from build123d import *

# Parameters (mm, degrees)
SKETCH_W        = 193
SKETCH_H        = 50
PAD_DEPTH       = 1.5
SKETCH001_W     = 193
SKETCH001_H     = 50
SKETCH001_W_2   = 190
SKETCH001_H_2   = 47.5
PAD001_DEPTH    = 28.5
SKETCH002_W     = 8
SKETCH002_H     = 6.75
PAD002_DEPTH    = 2
SKETCH003_R     = 3
PAD003_DEPTH    = 14.5
SKETCH004_R     = 2
POCKET_DEPTH    = 5
SKETCH005_W     = 13.4
SKETCH005_H     = 12
POCKET001_DEPTH = 5


with BuildPart() as part:
    # Sketch → Pad (new body)
    with BuildSketch(Plane.XY):
        with Locations((96.5, 25)):
            Rectangle(SKETCH_W, SKETCH_H)
    extrude(amount=PAD_DEPTH)

    # Sketch001 (on Face6 of Pad) → Pad001 (join)
    with BuildSketch(Plane.XY.offset(1.5)):
        with Locations((96.5, 25)):
            Rectangle(SKETCH001_W, SKETCH001_H)
        with Locations((96.5, 25)):
            Rectangle(SKETCH001_W_2, SKETCH001_H_2, mode=Mode.SUBTRACT)
    extrude(amount=PAD001_DEPTH)

    # Sketch002 (on Face15 of Pad001) → Pad002 (join)
    with BuildSketch(Plane.XY.offset(1.5)):
        with Locations((5.5, 45.375)):
            Rectangle(SKETCH002_W, SKETCH002_H)
        with Locations((187.5, 45.375)):
            Rectangle(SKETCH002_W, SKETCH002_H)
        with Locations((187.5, 4.625)):
            Rectangle(SKETCH002_W, SKETCH002_H)
        with Locations((5.5, 4.625)):
            Rectangle(SKETCH002_W, SKETCH002_H)
    extrude(amount=PAD002_DEPTH)

    # Sketch003 (on Face19 of Pad002) → Pad003 (join)
    with BuildSketch(Plane.XY.offset(3.5)):
        with Locations((5.5, 46)):
            Circle(SKETCH003_R)
        with Locations((5.5, 4)):
            Circle(SKETCH003_R)
        with Locations((187.5, 46)):
            Circle(SKETCH003_R)
        with Locations((187.5, 4)):
            Circle(SKETCH003_R)
    extrude(amount=PAD003_DEPTH)

    # Sketch004 (on Face24 of Pad003) → Pocket (cut)
    with BuildSketch(Plane.XY.offset(18)):
        with Locations((187.5, 46)):
            Circle(SKETCH004_R)
        with Locations((187.5, 4)):
            Circle(SKETCH004_R)
        with Locations((5.5, 46)):
            Circle(SKETCH004_R)
        with Locations((5.5, 4)):
            Circle(SKETCH004_R)
    extrude(amount=-POCKET_DEPTH, mode=Mode.SUBTRACT)

    # Sketch005 (on Face7 of Pocket) → Pocket001 (cut)
    with BuildSketch(Plane(origin=(0, 0, 0), x_dir=(0, -1, 0), z_dir=(-1, 0, 0))):
        with Locations((-25, 13.5)):
            Rectangle(SKETCH005_W, SKETCH005_H)
    extrude(amount=-POCKET001_DEPTH, mode=Mode.SUBTRACT)


solid = part.part
The model under review builds one solid part; all positions refer to its coordinate system, in mm. A direction names the side the tool comes from. Round coordinates to 2 decimals unless told otherwise and drop trailing zeros. Order: outer loops, then holes, each group sorted by start corner. A loop starts at its lowest first (then second) coordinate and runs counter-clockwise, first axis right, second up. Notation, with made-up numbers: (64, 4) -> (112, 4) arc R24 ccw to (112, 28) -> close; hole circle Ø11 at (27.25, -7.75). An arc over 180 degrees is marked (long way). Return JSON: item names as keys, results as strings.
1. Take a section at B-B (x = 131). Write out the cut boundary in (y, z), then the cut area to 3 significant figures.
Answer block:
{"outline": "(0, 0) -> (50, 0) -> (50, 30) -> (48.75, 30) -> (48.75, 1.5) -> (1.25, 1.5) -> (1.25, 30) -> (0, 30) -> close", "area": "146 mm²"}
2. For L1, parallel to Y at x = 187.5, z = 16.15; L2, parallel to Y at x = 83, z = 5, list the stretches that pass through material, from the lowest coordinate up. Write a range as [from, to].
Answer block:
{"L1": "y = [0, 2], [6, 7], [43, 44], [48, 50]", "L2": "y = [0, 1.25], [48.75, 50]"}
3. Take a section at A-A (y = 25). Write out the cut boundary in (x, z), then the cut area to 3 significant figures.
Answer block:
{"outline": "(0, 0) -> (193, 0) -> (193, 30) -> (191.5, 30) -> (191.5, 1.5) -> (1.5, 1.5) -> (1.5, 7.5) -> (0, 7.5) -> close; (0, 19.5) -> (1.5, 19.5) -> (1.5, 30) -> (0, 30) -> close", "area": "357 mm²"}
4. The part is to be moulded in two halves that separate along X. For faces 1 (the face through (96, 1, 30)), 2 (the face through (185, 46, 18)), 3 (the face through (0, 25, 21)), say which applies: +X half, -X half, draft (parallel to the pull), parting line (faces both ways), or undercut.
Answer block:
{"face 1": "draft", "face 2": "undercut", "face 3": "-X half"}
5. Take a section at D-D (y = 11). Write out the cut boundary in (x, z), then the cut area to 3 significant figures.
Answer block:
{"outline": "(0, 0) -> (193, 0) -> (193, 30) -> (191.5, 30) -> (191.5, 1.5) -> (1.5, 1.5) -> (1.5, 30) -> (0, 30) -> close", "area": "375 mm²"}
6. For faces 4 (the face through (4, 43, 3.5)), 5 (the face through (95, 25, 0)), list the 3-axis set-ups (+Z, -Z, +X, -X, +Y, -Y) from which the entire face can be reached by the end or side of a thin tool; tool diameter is ignored.
Answer block:
{"face 4": "+Z", "face 5": "-Z, +X, -X, +Y, -Y"}
7. Take a section at C-C (y = 46). Write out the cut boundary in (x, z).
Answer block:
{"outline": "(0, 0) -> (193, 0) -> (193, 30) -> (191.5, 30) -> (191.5, 3.5) -> (190.5, 3.5) -> (190.5, 18) -> (189.5, 18) -> (189.5, 13) -> (185.5, 13) -> (185.5, 18) -> (184.5, 18) -> (184.5, 3.5) -> (183.5, 3.5) -> (183.5, 1.5) -> (9.5, 1.5) -> (9.5, 3.5) -> (8.5, 3.5) -> (8.5, 18) -> (7.5, 18) -> (7.5, 13) -> (3.5, 13) -> (3.5, 18) -> (2.5, 18) -> (2.5, 3.5) -> (1.5, 3.5) -> (1.5, 30) -> (0, 30) -> close"}
8. Insertion check: P1, Ø5, axis at x = 30.5, y = 25.5, coming from the +Z side; P2, Ø1.7, axis at x = 186.5, y = 5, coming from the +Z side; P3, Ø1.2, axis at x = 5, y = 46.5, coming from the +Z side. Each pin has a flat end and moves straight along its axis. Give the tip position at first contact, or say it passes through.
Answer block:
{"P1": "stops at z = 1.5", "P2": "stops at z = 18", "P3": "stops at z = 13"}
